```python
from build123d import *
from build123d.topology import SkipClean

# Parameters (mm, degrees)
BOSS_EXTRUDE1_DEPTH = 44
SKETCH8_R           = 1.75
CUT_EXTRUDE1_DEPTH  = 7
SKETCH9_R           = 1.75
CUT_EXTRUDE2_DEPTH  = 7
CUT_EXTRUDE3_START  = 7
SKETCH10_R          = 1.75
CUT_EXTRUDE3_DEPTH  = 7
CUT_EXTRUDE4_START  = 7
SKETCH11_R          = 1.75
CUT_EXTRUDE4_DEPTH  = 7


with BuildPart() as part:
    # Sketch1 → Boss-Extrude1 (new body)
    with BuildSketch(Plane.XY):
        Polygon((-22, 15), (-22, 11), (-15, 11), (-15, 0), (-9, 0), (-9, 11), (9, 11), (9, 0), (15, 0), (15, 11), (22, 11), (22, 15), align=None)
    extrude(amount=BOSS_EXTRUDE1_DEPTH)

    # Sketch2 → Cut-Revolve1 (revolve, cut)
    with BuildSketch(Plane.XY.offset(5), mode=Mode.PRIVATE) as cut_revolve1_sk:
        Polygon((18.5, 15), (20, 15), (19.7295, 14.7295), (19.7295, 11.2705), (20, 11), (18.5, 11), align=None)
    revolve(cut_revolve1_sk.sketch.rotate(Axis((18.5, 11, 5), (0, 1, 0)), 270), axis=Axis((18.5, 11, 5), (0, 1, 0)), mode=Mode.SUBTRACT)

    # Sketch3 → Cut-Revolve2 (revolve, cut)
    with BuildSketch(Plane.XY.offset(39), mode=Mode.PRIVATE) as cut_revolve2_sk:
        Polygon((18.5, 15), (20, 15), (19.7295, 14.7295), (19.7295, 11.2705), (20, 11), (18.5, 11), align=None)
    revolve(cut_revolve2_sk.sketch.rotate(Axis((18.5, 11, 39), (0, 1, 0)), 270), axis=Axis((18.5, 11, 39), (0, 1, 0)), mode=Mode.SUBTRACT)

    # Sketch4 → Revolve1 (revolve)
    with SkipClean():  # the faces are left unmerged after this step: merging them gives an invalid solid
        with BuildSketch(Plane.XY.offset(10)):
            with BuildLine():
                Line((-10.07, 1.95), (-10.07, 8.05))
                ThreePointArc((-10.07, 8.05), (-7.02, 5), (-10.07, 1.95))
            make_face()
        revolve(axis=Axis((-10.07, -50, 10), (0, 1, 0)))

    # Sketch5 → Revolve2 (revolve)
    with SkipClean():  # the faces are left unmerged after this step: merging them gives an invalid solid
        with BuildSketch(Plane.XY.offset(34)):
            with BuildLine():
                Line((-10.07, 1.95), (-10.07, 8.05))
                ThreePointArc((-10.07, 8.05), (-7.02, 5), (-10.07, 1.95))
            make_face()
        revolve(axis=Axis((-10.07, -50, 34), (0, 1, 0)))

    # Sketch6 → Revolve3 (revolve)
    with SkipClean():  # the faces are left unmerged after this step: merging them gives an invalid solid
        with BuildSketch(Plane.XY.offset(34)):
            with BuildLine():
                Line((10.07, 8.05), (10.07, 1.95))
                ThreePointArc((10.07, 1.95), (7.02, 5), (10.07, 8.05))
            make_face()
        revolve(axis=Axis((10.07, 50, 34), (0, -1, 0)))

    # Sketch7 → Revolve4 (revolve)
    with SkipClean():  # the faces are left unmerged after this step: merging them gives an invalid solid
        with BuildSketch(Plane.XY.offset(10)):
            with BuildLine():
                Line((10.07, 8.05), (10.07, 1.95))
                ThreePointArc((10.07, 1.95), (7.02, 5), (10.07, 8.05))
            make_face()
        revolve(axis=Axis((10.07, 50, 10), (0, -1, 0)))

    # Sketch8 → Cut-Extrude1 (cut)
    with SkipClean():  # the faces are left unmerged after this step: merging them gives an invalid solid
        with BuildSketch(Plane(origin=(20.5, 0, 0), x_dir=(0, 0, -1), z_dir=(1, 0, 0))):
            with Locations((-10, 5)):
                Circle(SKETCH8_R)
        extrude(amount=-CUT_EXTRUDE1_DEPTH, mode=Mode.SUBTRACT)

    # Sketch9 → Cut-Extrude2 (cut)
    with SkipClean():  # the faces are left unmerged after this step: merging them gives an invalid solid
        with BuildSketch(Plane(origin=(20.5, 0, 0), x_dir=(0, 0, -1), z_dir=(1, 0, 0))):
            with Locations((-34, 5)):
                Circle(SKETCH9_R)
        extrude(amount=-CUT_EXTRUDE2_DEPTH, mode=Mode.SUBTRACT)

    # Sketch10 → Cut-Extrude3 (cut)
    with SkipClean():  # the faces are left unmerged after this step: merging them gives an invalid solid
        with BuildSketch(Plane(origin=(-20.5, 0, 0), x_dir=(0, 0, -1), z_dir=(1, 0, 0)).offset(CUT_EXTRUDE3_START)):
            with Locations((-10, 5)):
                Circle(SKETCH10_R)
        extrude(amount=-CUT_EXTRUDE3_DEPTH, mode=Mode.SUBTRACT)

    # Sketch11 → Cut-Extrude4 (cut)
    with SkipClean():  # the faces are left unmerged after this step: merging them gives an invalid solid
        with BuildSketch(Plane(origin=(-20.5, 0, 0), x_dir=(0, 0, -1), z_dir=(1, 0, 0)).offset(CUT_EXTRUDE4_START)):
            with Locations((-34, 5)):
                Circle(SKETCH11_R)
        extrude(amount=-CUT_EXTRUDE4_DEPTH, mode=Mode.SUBTRACT)

    # Sketch12 → Cut-Revolve3 (revolve, cut)
    with SkipClean():  # the faces are left unmerged after this step: merging them gives an invalid solid
        with BuildSketch(Plane.XY.offset(5), mode=Mode.PRIVATE) as cut_revolve3_sk:
            Polygon((-18.5, 15), (-17, 15), (-17.2705, 14.7295), (-17.2705, 11.2705), (-17, 11), (-18.5, 11), align=None)
        revolve(cut_revolve3_sk.sketch.rotate(Axis((-18.5, 11, 5), (0, 1, 0)), 270), axis=Axis((-18.5, 11, 5), (0, 1, 0)), mode=Mode.SUBTRACT)

    # Sketch13 → Cut-Revolve4 (revolve, cut)
    with SkipClean():  # the faces are left unmerged after this step: merging them gives an invalid solid
        with BuildSketch(Plane.XY.offset(39), mode=Mode.PRIVATE) as cut_revolve4_sk:
            Polygon((-18.5, 15), (-17, 15), (-17.2705, 14.7295), (-17.2705, 11.2705), (-17, 11), (-18.5, 11), align=None)
        revolve(cut_revolve4_sk.sketch.rotate(Axis((-18.5, 11, 39), (0, 1, 0)), 270), axis=Axis((-18.5, 11, 39), (0, 1, 0)), mode=Mode.SUBTRACT)

    # Sketch14 → Cut-Revolve5 (revolve, cut)
    with SkipClean():  # the faces are left unmerged after this step: merging them gives an invalid solid
        with BuildSketch(Plane(origin=(11.5, 0, 0), x_dir=(0, 0, -1), z_dir=(1, 0, 0)), mode=Mode.PRIVATE) as cut_revolve5_sk:
            Polygon((-11.5, 3.864115214), (-13.121, 4.8), (-13.121, 11.621), (-13.5, 12), (-14.35, 12), (-14.35, 15), (-11.5, 15), align=None)
        revolve(cut_revolve5_sk.sketch.rotate(Axis((11.5, 15, 11.5), (0, -1, 0)), 180), axis=Axis((11.5, 15, 11.5), (0, -1, 0)), mode=Mode.SUBTRACT)

    # Sketch15 → Cut-Revolve6 (revolve, cut)
    with SkipClean():  # the faces are left unmerged after this step: merging them gives an invalid solid
        with BuildSketch(Plane(origin=(11.5, 0, 0), x_dir=(0, 0, -1), z_dir=(1, 0, 0)), mode=Mode.PRIVATE) as cut_revolve6_sk:
            Polygon((-32.5, 15), (-29.65, 15), (-29.65, 12), (-30.5, 12), (-30.879, 11.621), (-30.879, 4.8), (-32.5, 3.864115214), align=None)
        revolve(cut_revolve6_sk.sketch.rotate(Axis((11.5, 3.864115214, 32.5), (0, 1, 0)), 180), axis=Axis((11.5, 3.864115214, 32.5), (0, 1, 0)), mode=Mode.SUBTRACT)

    # Sketch16 → Cut-Revolve7 (revolve, cut)
    with SkipClean():  # the faces are left unmerged after this step: merging them gives an invalid solid
        with BuildSketch(Plane(origin=(-11.5, 0, 0), x_dir=(0, 0, -1), z_dir=(1, 0, 0)), mode=Mode.PRIVATE) as cut_revolve7_sk:
            Polygon((-11.5, 3.864115214), (-13.121, 4.8), (-13.121, 11.621), (-13.5, 12), (-14.35, 12), (-14.35, 15), (-11.5, 15), align=None)
        revolve(cut_revolve7_sk.sketch.rotate(Axis((-11.5, 15, 11.5), (0, -1, 0)), 180), axis=Axis((-11.5, 15, 11.5), (0, -1, 0)), mode=Mode.SUBTRACT)

    # Sketch17 → Cut-Revolve8 (revolve, cut)
    with SkipClean():  # the faces are left unmerged after this step: merging them gives an invalid solid
        with BuildSketch(Plane(origin=(-11.5, 0, 0), x_dir=(0, 0, -1), z_dir=(1, 0, 0)), mode=Mode.PRIVATE) as cut_revolve8_sk:
            Polygon((-32.5, 15), (-29.65, 15), (-29.65, 12), (-30.5, 12), (-30.879, 11.621), (-30.879, 4.8), (-32.5, 3.864115214), align=None)
        revolve(cut_revolve8_sk.sketch.rotate(Axis((-11.5, 3.864115214, 32.5), (0, 1, 0)), 180), axis=Axis((-11.5, 3.864115214, 32.5), (0, 1, 0)), mode=Mode.SUBTRACT)


solid = part.part
```
For this review, take the finished solid that the model builds, in its own axes (mm). A direction names the side the tool comes from. Coordinates: 2 decimals unless noted, no trailing zeros. Order: outer loops, then holes, each group sorted by start corner. A loop starts at its lowest first (then second) coordinate and runs counter-clockwise, first axis right, second up. Notation, with made-up numbers: (-18, 39.5) -> (5, 39.5) arc R13 cw to (5, 53.5) -> close; hole circle Ø9 at (6, -21). An arc over 180 degrees is marked (long way). Use CSV: the item, a comma, the result in double quotes. Start each with the question number.
Item 1: For faces 1 (the face through (14.26, 3.45, 9.19)), 2 (the face through (-9.097, 13.479, 34.032)), 3 (the face through (-15, 6, 22)), 4 (the face through (-13.5, 5, 34)), list the 3-axis set-ups (+Z, -Z, +X, -X, +Y, -Y) from which the entire face can be reached by the end or side of a thin tool; tool diameter is ignored.
Item 2: Insertion check: pin 1 (5 mm diameter, centred on y = 4, z = 19.5, fed in from +X); pin 2 (5 mm diameter, centred on y = 3.5, z = 39.5, fed in from -X); pin 3 (5.5 mm diameter, centred on x = 18.5, z = 25, fed in from -Y). Each pin has a flat end and moves straight along its axis. Give the tip position at first contact, or say it passes through.
Item 3: Draft analysis for pull direction Y (two halves, no side actions). For faces 5 (the face through (9.6, 12, 12.7)), 6 (the face through (13.107, 8.258, 11.711)), 7 (the face through (14.26, 3.94, 35.39)), state which applies: pulls with the +Y half, pulls with the -Y half, needs draft (parallel to the pull), parting line crosses it, or undercut.
Item 4: We need section B-B, the plane z = 39. Give the boundary of the cut face in (x, y).
Item 5: We need section D-D, the plane y = 13.25. Give the number of separate pieces and of enclosed holes in the cut face, then the cut area to 3 significant figures.
Item 6: We need section C-C, the plane x = -18.5. Give the boundary of the cut face in (y, z).
Item 7: Wall thickness on probe 1 along X at (y, z) = (13.35, 32.5); probe 2 along X at (y, z) = (6.25, 17); probe 3 along X at (y, z) = (13.9, 39): over which ranges is each line inside the solid? List them lowest first.
Derived:
1,face 1,"+X"
1,face 2,"+Y"
1,face 3,"+Z, -Z, -X, -Y"
1,face 4,"-X"
2,pin 1,"stops at x = 15"
2,pin 2,"stops at x = -15"
2,pin 3,"stops at y = 11"
3,face 5,"pulls with the +Y half"
3,face 6,"needs draft"
3,face 7,"undercut"
4,outline,"(-22, 11) -> (-20, 11) -> (-19.73, 11.27) -> (-19.73, 14.73) -> (-20, 15) -> (-22, 15) -> close; (-17.27, 11.27) -> (-17, 11) -> (-15, 11) -> (-15, 0) -> (-9, 0) -> (-9, 11) -> (9, 11) -> (9, 0) -> (15, 0) -> (15, 11) -> (17, 11) -> (17.27, 11.27) -> (17.27, 14.73) -> (17, 15) -> (-17, 15) -> (-17.27, 14.73) -> close; (19.73, 11.27) -> (20, 11) -> (22, 11) -> (22, 15) -> (20, 15) -> (19.73, 14.73) -> close"
5,separate pieces,"1"
5,enclosed holes,"8"
5,area,"1,810 mm^2"
6,outline,"(11, 0) -> (15, 0) -> (15, 3.5) -> (14.73, 3.77) -> (11.27, 3.77) -> (11, 3.5) -> close; (11, 6.5) -> (11.27, 6.23) -> (14.73, 6.23) -> (15, 6.5) -> (15, 37.5) -> (14.73, 37.77) -> (11.27, 37.77) -> (11, 37.5) -> close; (11, 40.5) -> (11.27, 40.23) -> (14.73, 40.23) -> (15, 40.5) -> (15, 44) -> (11, 44) -> close"
7,probe 1,"x = -22 to -14.35, -8.65 to 8.65, 14.35 to 22"
7,probe 2,"x = -15 to -9, 9 to 15"
7,probe 3,"x = -22 to -19.73, -17.27 to 17.27, 19.73 to 22"
